```python
from build123d import *

# Parameters (mm, degrees)
SKETCH_2_W             = 28
SKETCH_2_H             = 4.5
CUT_EXTRUDE_1_DEPTH    = 10
EXTRUDE_1_DEPTH        = 15
HOLE_WIZARD_M3_1_D     = 2.5
HOLE_WIZARD_M3_1_DEPTH = 4
HOLE_WIZARD_M3_1_TIP   = 0.751075774
CUT_EXTRUDE_START      = -20
CUT_EXTRUDE_2_DEPTH    = 20
HOLE_WIZARD_M4_1_D     = 3.3
HOLE_WIZARD_M4_1_DEPTH = 10.1
HOLE_WIZARD_M4_1_TIP   = 0.991420021
HOLE_WIZARD_M3_2_D     = 2.5
HOLE_WIZARD_M5_1_D     = 4.2
HOLE_WIZARD_M5_1_DEPTH = 14
HOLE_WIZARD_M5_1_TIP   = 1.2618073


with BuildPart() as part:
    # 草图1 → 旋转1 (revolve)
    with BuildSketch(Plane.XY, mode=Mode.PRIVATE) as revolve_1_sk:
        Polygon((0, 0), (4.1, 0), (4.1, 6.7), (13.4, 6.7), (13.4, 8.7), (21, 8.7), (21, 10.2), (20, 10.2), (20, 11.2), (21, 11.2), (21, 12.2), (10, 12.2), (10, 13.2), (21, 13.2), (21, 20.4), (5, 20.4), (5, 21), (21, 21), (21, 34.7), (18.3, 38.7), (3.5, 38.7), (3.5, 43.7), (0, 43.7), align=None)
    revolve(revolve_1_sk.sketch.rotate(Axis((0, 43.7, 0), (0, -1, 0)), 90), axis=Axis((0, 43.7, 0), (0, -1, 0)))

    # 草图2 → 切除-拉伸1 (cut)
    with BuildSketch(Plane.XY.offset(21)):
        with Locations((0, 16.05)):
            Rectangle(SKETCH_2_W, SKETCH_2_H)
    extrude(amount=-CUT_EXTRUDE_1_DEPTH, mode=Mode.SUBTRACT)

    # 草图3 → 凸台-拉伸1 (add)
    with BuildSketch(Plane.XY.offset(11)):
        with BuildLine():
            Line((9.185056323, 18.053194417), (9.385056323, 18.053194417))
            ThreePointArc((9.385056323, 18.053194417), (11.385056323, 16.053194417), (9.385056323, 14.053194417))
            Line((9.385056323, 14.053194417), (9.185056323, 14.053194417))
            ThreePointArc((9.185056323, 14.053194417), (7.185056323, 16.053194417), (9.185056323, 18.053194417))
        make_face()
    extrude(amount=EXTRUDE_1_DEPTH)

    # M3 螺纹孔1
    with Locations(Plane(origin=(0, 38.7, 0), x_dir=(1, 0, 0), z_dir=(0, 1, 0))):
        with Locations((-6.5, 0), (6.5, 0)):
            Hole(HOLE_WIZARD_M3_1_D / 2, depth=HOLE_WIZARD_M3_1_DEPTH)
            with Locations((0, 0, -(HOLE_WIZARD_M3_1_DEPTH + HOLE_WIZARD_M3_1_TIP / 2))):  # 118° drill point
                Cone(0, HOLE_WIZARD_M3_1_D / 2, HOLE_WIZARD_M3_1_TIP, mode=Mode.SUBTRACT)

    # 草图7 → 旋转2 (revolve)
    with BuildSketch(Plane.XY, mode=Mode.PRIVATE) as revolve_2_sk:
        Polygon((0, -54.6), (5, -54.6), (5, -30.5), (8.275, -30.5), (8.275, -29.6), (13, -29.6), (13, -27.6), (21, -27.6), (21, 8.7), (0, 8.7), align=None)
    revolve(revolve_2_sk.sketch.rotate(Axis((0, 8.7, 0), (0, -1, 0)), 180), axis=Axis((0, 8.7, 0), (0, -1, 0)))

    # 草图8 → 切除-拉伸2 (cut)
    with BuildSketch(Plane.XZ.offset(54.6).offset(CUT_EXTRUDE_START)):
        with BuildLine():
            Line((-3, 4), (3, 4))
            ThreePointArc((3, 4), (0, 5), (-3, 4))
        make_face()
    extrude(amount=CUT_EXTRUDE_2_DEPTH, mode=Mode.SUBTRACT)

    # M4 螺纹孔1
    with Locations(Plane(origin=(0, -27.6, 0), x_dir=(-1, 0, 0), z_dir=(0, -1, 0))):
        with Locations((0, -17.5), (-17.5, 0), (0, 17.5), (17.5, 0)):
            Hole(HOLE_WIZARD_M4_1_D / 2, depth=HOLE_WIZARD_M4_1_DEPTH)
            with Locations((0, 0, -(HOLE_WIZARD_M4_1_DEPTH + HOLE_WIZARD_M4_1_TIP / 2))):  # 118° drill point
                Cone(0, HOLE_WIZARD_M4_1_D / 2, HOLE_WIZARD_M4_1_TIP, mode=Mode.SUBTRACT)

    # M3 螺纹孔2 (through all)
    with Locations(Plane(origin=(0, -44.6, 4), x_dir=(1, 0, 0), z_dir=(0, 0, 1))):
        with Locations((0, 0)):
            Hole(HOLE_WIZARD_M3_2_D / 2)

    # M5 螺纹孔1
    with Locations(Plane(origin=(0, -54.6, 0), x_dir=(-1, 0, 0), z_dir=(0, -1, 0))):
        with Locations((0, 0)):
            Hole(HOLE_WIZARD_M5_1_D / 2, depth=HOLE_WIZARD_M5_1_DEPTH)
            with Locations((0, 0, -(HOLE_WIZARD_M5_1_DEPTH + HOLE_WIZARD_M5_1_TIP / 2))):  # 118° drill point
                Cone(0, HOLE_WIZARD_M5_1_D / 2, HOLE_WIZARD_M5_1_TIP, mode=Mode.SUBTRACT)


solid = part.part
```
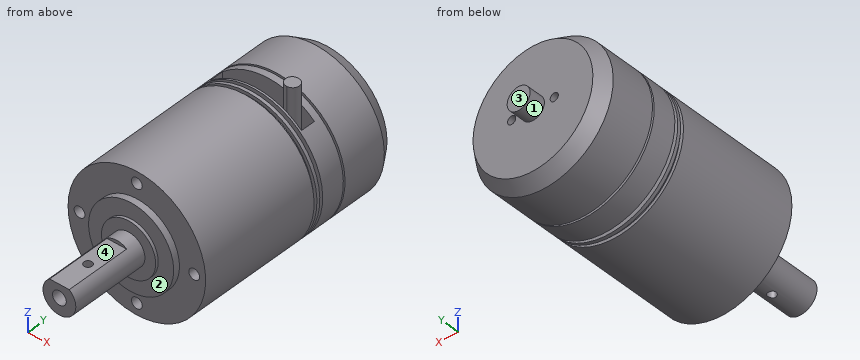
CAD build for the part. Positions are in the model's coordinates, mm. Face numbers are marked on the shaded views. A direction names the side the tool comes from. Give positions to 0.01 mm unless a question says otherwise; leave off trailing zeros. Loops run counter-clockwise (first coordinate to the right, second up) from the corner with the lowest first, then second, coordinate; pieces in that order, holes last. Notation, with made-up numbers: M 34.25,-16 L 64.25,-16 A16 ccw 64.25,6 Z; hole C -16,67 d11. An arc over 180 degrees is marked long. Use one line per item in the form item = value.
Item 1: Flat gauge pins, fed straight in: pin 1 (4 mm diameter, centred on y = -28.5, z = 9, fed in from -X); pin 2 (4.5 mm diameter, centred on x = -17.5, z = 0, fed in from -Y); pin 3 (8 mm diameter, centred on x = -4, z = 15, fed in from -Y). Where does each tip first touch, or does it go through?
Determined:
pin_1 = -19.72
pin_2 = -27.6
pin_3 = -29.6
Item 2: Slice it at D-D (y = 3). List the corners of the cut face in (x, z), plus the area to 3 significant figures.
Determined:
outline = C 0,0 d42
area = 1,390 mm2
Item 3: Slice it at A-A (y = -44.6). List the corners of the cut face in (x, z).
Determined:
outline = M -3,4 A5 ccw -1.25,-4.84 L -1.25,-1.69 A2.1 cw -1.25,1.69 L -1.25,4 Z; M 1.25,-4.84 A5 ccw 3,4 L 1.25,4 L 1.25,1.69 A2.1 cw 1.25,-1.69 Z
Item 4: Slice it at B-B (z = -14.5). Count the separate pieces of the cut face and the enclosed holes in it, plus the area to 3 significant figures.
Determined:
separate_pieces = 3
enclosed_holes = 0
area = 1,950 mm2
Item 5: Which spindle directions (+Z, -Z, +X, -X, +Y, -Y) get a long thin tool onto all of the face, cutting with end or side? Do the marked faces 1, 2, 3 and 4. Say none if no direction does.
Determined:
face_1 = +Y
face_2 = -Y
face_3 = +Z, -Z, +X, -X, +Y
face_4 = +Z, +X, -X, -Y
Item 6: Drill centre lines: probe 1 along Y at (x, z) = (-2.5, 16.5); probe 2 along Y at (x, z) = (15, -10.5); probe 3 along Y at (x, z) = (-10, 7.5). Where is each one in solid material? Low to high. Write a range as from..to.
Determined:
probe_1 = -27.6..12.2, 13.2..13.8, 18.3..20.4, 21..38.7
probe_2 = -27.6..12.2, 13.2..20.4, 21..38.69
probe_3 = -29.6..12.2, 13.2..20.4, 21..38.7
